Geometry: final body of the model. Coordinates: model frame, mm. A direction names the side the tool comes from. Give positions to 0.01 mm unless a question says otherwise; leave off trailing zeros. Order: outer loops, then holes, each group sorted by start corner. A loop starts at its lowest first (then second) coordinate and runs counter-clockwise, first axis right, second up. Notation, with made-up numbers: (33, 58.5) -> (73, 58.5) arc R23 cw to (73, 81.5) -> close; hole circle Ø10 at (-12, -5.75). An arc over 180 degrees is marked (long way). Answer in a Markdown table with one row per item. Add a question column.
Q1. Line query: line 1 along Y through (x, z) = (0, 29); line 2 along X through (y, z) = (-0.5, 1); line 3 along Y through (x, z) = (0, 10). Output: solid intervals per line, ascending. Write a range as from..to.
Q2. Cut plane D-D on y = -11.5. Return the cut outline in (x, z), and give its area (3 significant figures).
Q3. Cut plane A-A on y = 0. Return the cut outline in (x, z).
Q4. Cut plane C-C on z = 9.5. Return the cut outline in (x, y).
Q5. Pull-direction query (Y, two-part tool) for faces 1 (the face through (-6, -12, 0)), 2 (the face through (-10.316, -7.91, 10.353)), 3 (the face through (-6.07, -27.334, 15.776)); classes: +Y half, -Y half, draft (parallel to the pull), parting line (faces both ways), or undercut.
Q6. Contact query for flat-ended pins moving along their axis: P1, Ø4, axis at x = 11, z = 8.5, coming from the +Y side; P2, Ø13, axis at x = -2, y = 2, coming from the -Z side; P3, Ø12, axis at x = -8, y = 21.5, coming from the -Z side; P4, Ø6, axis at x = -20.5, z = 17, coming from the -Y side. Output: stop coordinate, or through.
Q7. Set-up query: faces 4 (the face through (-3, 9, 21)), 5 (the face through (8.584, 2.703, 26.423)). Return all of +Z, -Z, +X, -X, +Y, -Y with unobstructed straight access to the full face (end or side cutting, diameter ignored); none if empty.
from build123d import *

# Parameters (mm, degrees)
SZKIC1_W                    = 32
SZKIC1_H                    = 28
SZKIC3_R                    = 21
DODANIE_WYCI_GNI_CIE1_DEPTH = 14


# Read off the part's stored shape, not the designer's step: Usuń ścianę1
with BuildPart() as part:
    # Szkic1 → Obrót1 (revolve)
    with BuildSketch(Plane(origin=(0, 0, 0), x_dir=(0, 0, -1), z_dir=(1, 0, 0)), mode=Mode.PRIVATE) as obr_t1_sk:
        with Locations((-16, 14)):
            Rectangle(SZKIC1_W, SZKIC1_H)
    revolve(obr_t1_sk.sketch.rotate(Axis((0, 0, 0), (0, 0, 1)), 270), axis=Axis((0, 0, 0), (0, 0, 1)))

    # Szkic2 → Wycięcie-obrót1 (revolve, cut)
    with BuildSketch(Plane(origin=(0, 0, 0), x_dir=(0, 0, -1), z_dir=(1, 0, 0)), mode=Mode.PRIVATE) as wyci_cie_obr_t1_sk:
        Polygon((-32, 0), (-32, 9), (-21, 9), (-21, 13), (0, 13), (0, 0), align=None)
    revolve(wyci_cie_obr_t1_sk.sketch.rotate(Axis((0, 0, 0), (0, 0, 1)), 270), axis=Axis((0, 0, 0), (0, 0, 1)), mode=Mode.SUBTRACT)


with BuildPart() as body_2:
    # Szkic3 → Dodanie-wyciągnięcie1 (new body)
    with BuildSketch(Plane(origin=(0, 0, 0), x_dir=(0, 0, -1), z_dir=(1, 0, 0))):
        Circle(SZKIC3_R)
    extrude(amount=DODANIE_WYCI_GNI_CIE1_DEPTH)


solid = part.part
Completed:
| question | item | result |
|---|---|---|
| 1 | line 1 | y = -28..-9, 9..28 |
| 1 | line 2 | x = -28..-12.99, 12.99..28 |
| 1 | line 3 | y = -28..-13, 13..28 |
| 2 | outline | (-25.53, 0) -> (-6.06, 0) -> (-6.06, 21) -> (6.06, 21) -> (6.06, 0) -> (25.53, 0) -> (25.53, 32) -> (-25.53, 32) -> close |
| 2 | area | 1,380 mm² |
| 3 | outline | (-28, 0) -> (-13, 0) -> (-13, 21) -> (-9, 21) -> (-9, 32) -> (-28, 32) -> close; (9, 21) -> (13, 21) -> (13, 0) -> (28, 0) -> (28, 32) -> (9, 32) -> close |
| 4 | outline | circle Ø56 at (0, 0); hole circle Ø26 at (0, 0) |
| 5 | face 1 | draft |
| 5 | face 2 | undercut |
| 5 | face 3 | parting line |
| 6 | P1 | stops at y = 26.51 |
| 6 | P2 | stops at z = 21 |
| 6 | P3 | stops at z = 0 |
| 6 | P4 | stops at y = -21.86 |
| 7 | face 4 | -Z |
| 7 | face 5 | +Z, -Z |
